from build123d import *

# Parameters (mm, degrees)
ESQUISSE2_W             = 50
ESQUISSE2_H             = 40
BOSS_EXTRU_1_DEPTH      = 5
ESQUISSE3_W             = 73
ESQUISSE3_H             = 38
BOSS_EXTRU_2_DEPTH      = 2.5
ENL_V_MAT_EXTRU_1_REACH = 64.75
ESQUISSE4_R             = 2
ENL_V_MAT_EXTRU_2_REACH = 64.75
ESQUISSE5_W             = 7
ESQUISSE5_H             = 15
CONG_1_R                = 2
CONG_2_R                = 5
CONG_3_R                = 2
ENL_V_MAT_EXTRU_3_DEPTH = 2
ENL_V_MAT_EXTRU_4_REACH = 64.107
ESQUISSE7_R             = 3.5
ENL_V_MAT_EXTRU_5_REACH = 61.643
ESQUISSE8_R             = 2


with BuildPart() as part:
    # Esquisse2 → Boss.-Extru.1 (new body)
    with BuildSketch(Plane(origin=(0, 0, 0), x_dir=(1, 0, 0), z_dir=(0, 1, 0))):
        Rectangle(ESQUISSE2_W, ESQUISSE2_H)
    extrude(amount=BOSS_EXTRU_1_DEPTH)

    # Esquisse3 → Boss.-Extru.2 (add, symmetric)
    with BuildSketch(Plane(origin=(0, 0, 0), x_dir=(0, 0, -1), z_dir=(1, 0, 0))):
        with Locations((0, 24)):
            Rectangle(ESQUISSE3_W, ESQUISSE3_H)
    extrude(amount=BOSS_EXTRU_2_DEPTH, both=True)

    # Esquisse4 → Enl_v. mat.-Extru.1 (cut, up to next)
    with BuildSketch(Plane(origin=(2.5, 0, 0), x_dir=(0, 0, -1), z_dir=(1, 0, 0)), mode=Mode.PRIVATE) as enl_v_mat_extru_1_sk1:
        with Locations((-27.94, 37.97)):
            Circle(ESQUISSE4_R)
    enl_v_mat_extru_1_tool1 = extrude(enl_v_mat_extru_1_sk1.sketch, amount=-ENL_V_MAT_EXTRU_1_REACH, mode=Mode.PRIVATE) & part.part
    # Esquisse4 → Enl_v. mat.-Extru.1 (cut, up to next)
    with BuildSketch(Plane(origin=(2.5, 0, 0), x_dir=(0, 0, -1), z_dir=(1, 0, 0)), mode=Mode.PRIVATE) as enl_v_mat_extru_1_sk2:
        with Locations((-27.94, 10.03)):
            Circle(ESQUISSE4_R)
    enl_v_mat_extru_1_tool2 = extrude(enl_v_mat_extru_1_sk2.sketch, amount=-ENL_V_MAT_EXTRU_1_REACH, mode=Mode.PRIVATE) & part.part
    # Esquisse4 → Enl_v. mat.-Extru.1 (cut, up to next)
    with BuildSketch(Plane(origin=(2.5, 0, 0), x_dir=(0, 0, -1), z_dir=(1, 0, 0)), mode=Mode.PRIVATE) as enl_v_mat_extru_1_sk3:
        with Locations((27.94, 37.97)):
            Circle(ESQUISSE4_R)
    enl_v_mat_extru_1_tool3 = extrude(enl_v_mat_extru_1_sk3.sketch, amount=-ENL_V_MAT_EXTRU_1_REACH, mode=Mode.PRIVATE) & part.part
    # Esquisse4 → Enl_v. mat.-Extru.1 (cut, up to next)
    with BuildSketch(Plane(origin=(2.5, 0, 0), x_dir=(0, 0, -1), z_dir=(1, 0, 0)), mode=Mode.PRIVATE) as enl_v_mat_extru_1_sk4:
        with Locations((27.94, 10.03)):
            Circle(ESQUISSE4_R)
    enl_v_mat_extru_1_tool4 = extrude(enl_v_mat_extru_1_sk4.sketch, amount=-ENL_V_MAT_EXTRU_1_REACH, mode=Mode.PRIVATE) & part.part
    add(enl_v_mat_extru_1_tool1.solids().sort_by_distance((2.5, 37.97, 27.94))[0], mode=Mode.SUBTRACT)
    add(enl_v_mat_extru_1_tool2.solids().sort_by_distance((2.5, 10.03, 27.94))[0], mode=Mode.SUBTRACT)
    add(enl_v_mat_extru_1_tool3.solids().sort_by_distance((2.5, 37.97, -27.94))[0], mode=Mode.SUBTRACT)
    add(enl_v_mat_extru_1_tool4.solids().sort_by_distance((2.5, 10.03, -27.94))[0], mode=Mode.SUBTRACT)

    # Esquisse5 → Enl_v. mat.-Extru.2 (cut, up to next)
    with BuildSketch(Plane(origin=(2.5, 0, 0), x_dir=(0, 0, -1), z_dir=(1, 0, 0)), mode=Mode.PRIVATE) as enl_v_mat_extru_2_sk1:
        with Locations((-33, 24)):
            Rectangle(ESQUISSE5_W, ESQUISSE5_H)
    enl_v_mat_extru_2_tool1 = extrude(enl_v_mat_extru_2_sk1.sketch, amount=-ENL_V_MAT_EXTRU_2_REACH, mode=Mode.PRIVATE) & part.part
    # Esquisse5 → Enl_v. mat.-Extru.2 (cut, up to next)
    with BuildSketch(Plane(origin=(2.5, 0, 0), x_dir=(0, 0, -1), z_dir=(1, 0, 0)), mode=Mode.PRIVATE) as enl_v_mat_extru_2_sk2:
        with Locations((33, 24)):
            Rectangle(ESQUISSE5_W, ESQUISSE5_H)
    enl_v_mat_extru_2_tool2 = extrude(enl_v_mat_extru_2_sk2.sketch, amount=-ENL_V_MAT_EXTRU_2_REACH, mode=Mode.PRIVATE) & part.part
    add(enl_v_mat_extru_2_tool1.solids().sort_by_distance((2.5, 24, 33))[0], mode=Mode.SUBTRACT)
    add(enl_v_mat_extru_2_tool2.solids().sort_by_distance((2.5, 24, -33))[0], mode=Mode.SUBTRACT)

    # Cong_1
    cong_1_edges = [part.edges().sort_by_distance(p)[0] for p in [
        (0, 16.5, -29.5),
        (0, 31.5, -29.5),
        (0, 16.5, 29.5),
        (0, 31.5, 29.5),
        (-2.5, 5, 0),
        (2.5, 5, 0),
    ]]
    fillet(cong_1_edges, radius=CONG_1_R)
    cong_1_2_edges = [part.edges().sort_by_distance(p)[0] for p in [
        (0, 5, -36.5),
        (0, 16.5, -36.5),
        (0, 43, -36.5),
        (0, 31.5, -36.5),
        (0, 5, 36.5),
        (0, 16.5, 36.5),
        (0, 31.5, 36.5),
        (0, 43, 36.5),
    ]]
    fillet(cong_1_2_edges, radius=CONG_1_R)

    # Cong_2
    cong_2_edges = [part.edges().sort_by_distance(p)[0] for p in [
        (25, 2.5, 20),
        (-25, 2.5, 20),
        (-25, 2.5, -20),
        (25, 2.5, -20),
    ]]
    fillet(cong_2_edges, radius=CONG_2_R)

    # Cong_3
    cong_3_edges = [part.edges().sort_by_distance(p)[0] for p in [
        (-2.5, 6, 20),
        (2.5, 6, 20),
        (0, 5, 20),
        (2.5, 6, -20),
        (-2.5, 6, -20),
        (0, 5, -20),
    ]]
    fillet(cong_3_edges, radius=CONG_3_R - 0.0001)  # a hair under: the kernel refuses the full size

    # Esquisse6 → Enl_v. mat.-Extru.3 (cut)
    with BuildSketch(Plane(origin=(0, 5, 0), x_dir=(1, 0, 0), z_dir=(0, 1, 0))):
        Polygon((-12.113248654, 10), (-13.556624327, 12.5), (-16.443375673, 12.5), (-17.886751346, 10), (-16.443375673, 7.5), (-13.556624327, 7.5), align=None)
        Polygon((-12.113248654, -10), (-13.556624327, -7.5), (-16.443375673, -7.5), (-17.886751346, -10), (-16.443375673, -12.5), (-13.556624327, -12.5), align=None)
        Polygon((13.556624327, -12.5), (12.113248654, -10), (13.556624327, -7.5), (16.443375673, -7.5), (17.886751346, -10), (16.443375673, -12.5), align=None)
        Polygon((13.556624327, 7.5), (12.113248654, 10), (13.556624327, 12.5), (16.443375673, 12.5), (17.886751346, 10), (16.443375673, 7.5), align=None)
    extrude(amount=-ENL_V_MAT_EXTRU_3_DEPTH, mode=Mode.SUBTRACT)

    # Esquisse7 → Enl_v. mat.-Extru.4 (cut, up to next)
    with BuildSketch(Plane.ZY.offset(1), mode=Mode.PRIVATE) as enl_v_mat_extru_4_sk1:
        with Locations((-27.94, 37.97)):
            Circle(ESQUISSE7_R)
    enl_v_mat_extru_4_tool1 = extrude(enl_v_mat_extru_4_sk1.sketch, amount=ENL_V_MAT_EXTRU_4_REACH, mode=Mode.PRIVATE) & part.part
    # Esquisse7 → Enl_v. mat.-Extru.4 (cut, up to next)
    with BuildSketch(Plane.ZY.offset(1), mode=Mode.PRIVATE) as enl_v_mat_extru_4_sk2:
        with Locations((-27.94, 10.03)):
            Circle(ESQUISSE7_R)
    enl_v_mat_extru_4_tool2 = extrude(enl_v_mat_extru_4_sk2.sketch, amount=ENL_V_MAT_EXTRU_4_REACH, mode=Mode.PRIVATE) & part.part
    # Esquisse7 → Enl_v. mat.-Extru.4 (cut, up to next)
    with BuildSketch(Plane.ZY.offset(1), mode=Mode.PRIVATE) as enl_v_mat_extru_4_sk3:
        with Locations((27.94, 37.97)):
            Circle(ESQUISSE7_R)
    enl_v_mat_extru_4_tool3 = extrude(enl_v_mat_extru_4_sk3.sketch, amount=ENL_V_MAT_EXTRU_4_REACH, mode=Mode.PRIVATE) & part.part
    # Esquisse7 → Enl_v. mat.-Extru.4 (cut, up to next)
    with BuildSketch(Plane.ZY.offset(1), mode=Mode.PRIVATE) as enl_v_mat_extru_4_sk4:
        with Locations((27.94, 10.03)):
            Circle(ESQUISSE7_R)
    enl_v_mat_extru_4_tool4 = extrude(enl_v_mat_extru_4_sk4.sketch, amount=ENL_V_MAT_EXTRU_4_REACH, mode=Mode.PRIVATE) & part.part
    enl_v_mat_extru_4_1 = enl_v_mat_extru_4_tool1.solids().sort_by_distance((-1, 37.97, -27.94))[0]
    add(enl_v_mat_extru_4_1, mode=Mode.SUBTRACT)
    enl_v_mat_extru_4_2 = enl_v_mat_extru_4_tool2.solids().sort_by_distance((-1, 10.03, -27.94))[0]
    add(enl_v_mat_extru_4_2, mode=Mode.SUBTRACT)
    enl_v_mat_extru_4_3 = enl_v_mat_extru_4_tool3.solids().sort_by_distance((-1, 37.97, 27.94))[0]
    add(enl_v_mat_extru_4_3, mode=Mode.SUBTRACT)
    enl_v_mat_extru_4_4 = enl_v_mat_extru_4_tool4.solids().sort_by_distance((-1, 10.03, 27.94))[0]
    add(enl_v_mat_extru_4_4, mode=Mode.SUBTRACT)
    enl_v_mat_extru_4 = enl_v_mat_extru_4_1 + enl_v_mat_extru_4_2 + enl_v_mat_extru_4_3 + enl_v_mat_extru_4_4  # Enl_v. mat.-Extru.4 as one shape, for the pattern or mirror that repeats it

    # Sym_trie3: Enl_v. mat.-Extru.4 across plane
    add(enl_v_mat_extru_4.mirror(Plane(origin=(0, 0, 0), x_dir=(0, 0, 1), z_dir=(1, 0, 0))), mode=Mode.SUBTRACT)

    # Esquisse8 → Enl_v. mat.-Extru.5 (cut, up to next)
    with BuildSketch(Plane(origin=(0, 3, 0), x_dir=(1, 0, 0), z_dir=(0, 1, 0)), mode=Mode.PRIVATE) as enl_v_mat_extru_5_sk1:
        with Locations(Location((-15, 10, 0), (0, 0, 270))):
            Circle(ESQUISSE8_R)
    enl_v_mat_extru_5_tool1 = extrude(enl_v_mat_extru_5_sk1.sketch, amount=-ENL_V_MAT_EXTRU_5_REACH, mode=Mode.PRIVATE) & part.part
    # Esquisse8 → Enl_v. mat.-Extru.5 (cut, up to next)
    with BuildSketch(Plane(origin=(0, 3, 0), x_dir=(1, 0, 0), z_dir=(0, 1, 0)), mode=Mode.PRIVATE) as enl_v_mat_extru_5_sk2:
        with Locations(Location((-15, -10, 0), (0, 0, 270))):
            Circle(ESQUISSE8_R)
    enl_v_mat_extru_5_tool2 = extrude(enl_v_mat_extru_5_sk2.sketch, amount=-ENL_V_MAT_EXTRU_5_REACH, mode=Mode.PRIVATE) & part.part
    # Esquisse8 → Enl_v. mat.-Extru.5 (cut, up to next)
    with BuildSketch(Plane(origin=(0, 3, 0), x_dir=(1, 0, 0), z_dir=(0, 1, 0)), mode=Mode.PRIVATE) as enl_v_mat_extru_5_sk3:
        with Locations(Location((15, -10, 0), (0, 0, 270))):
            Circle(ESQUISSE8_R)
    enl_v_mat_extru_5_tool3 = extrude(enl_v_mat_extru_5_sk3.sketch, amount=-ENL_V_MAT_EXTRU_5_REACH, mode=Mode.PRIVATE) & part.part
    # Esquisse8 → Enl_v. mat.-Extru.5 (cut, up to next)
    with BuildSketch(Plane(origin=(0, 3, 0), x_dir=(1, 0, 0), z_dir=(0, 1, 0)), mode=Mode.PRIVATE) as enl_v_mat_extru_5_sk4:
        with Locations(Location((15, 10, 0), (0, 0, 270))):
            Circle(ESQUISSE8_R)
    enl_v_mat_extru_5_tool4 = extrude(enl_v_mat_extru_5_sk4.sketch, amount=-ENL_V_MAT_EXTRU_5_REACH, mode=Mode.PRIVATE) & part.part
    add(enl_v_mat_extru_5_tool1.solids().sort_by_distance((-15, 3, -10))[0], mode=Mode.SUBTRACT)
    add(enl_v_mat_extru_5_tool2.solids().sort_by_distance((-15, 3, 10))[0], mode=Mode.SUBTRACT)
    add(enl_v_mat_extru_5_tool3.solids().sort_by_distance((15, 3, 10))[0], mode=Mode.SUBTRACT)
    add(enl_v_mat_extru_5_tool4.solids().sort_by_distance((15, 3, -10))[0], mode=Mode.SUBTRACT)


solid = part.part
Could you check a few things on this model? Use its own coordinates, in mm. A direction names the side the tool comes from. Coordinates: 2 decimals unless noted, no trailing zeros. Order: outer loops, then holes, each group sorted by start corner. A loop starts at its lowest first (then second) coordinate and runs counter-clockwise, first axis right, second up. Notation, with made-up numbers: (-12.75, 50.5) - (31.25, 50.5) arc R27 ccw to (31.25, 76.5) - close; hole circle Ø3 at (51.5, 88). An arc over 180 degrees is marked (long way). Answer in a Markdown table with one row per item. Add a question column.
(1) I need wall thicknesses on L1, parallel to Y at x = 1.95, z = -27.94; L2, parallel to Z at x = 1.75, y = 37.97; L3, parallel to X at y = 2.3, z = -10. Which ranges of each line are inside material? Lowest first, please.
(2) If we section it at A-A, the plane x = 15: Please give me the cut outline in (y, z), then the cut area to 3 significant figures.
(3) If we section it at D-D, the plane z = 0.5: Please give me the cut outline in (x, y), then the cut area to 3 significant figures.
(4) Will these pins go through, and if not, where does the flat tip stop? pin 1 (2 mm diameter, centred on x = -15, y = 4, fed in from -Z); pin 2 (8 mm diameter, centred on x = -19.5, z = -18.5, fed in from +Y); pin 3 (6 mm diameter, centred on y = 16.5, z = -28, fed in from -X); pin 4 (3 mm diameter, centred on x = -9.5, z = 20, fed in from -Y).
(5) If we section it at B-B, the plane z = -27.94: Please give me the cut outline in (x, y).
(6) If we mould it in two halves opening along Y, with no side actions, what happens to faces 1 (the face through (0.06, 4.13, -20.35)), 2 (the face through (13, 3, 11)), 3 (the face through (1, 10.1, 30.2)), 4 (the face through (-13, 2, -10))? For each: released by +Y, released by -Y, zero draft, split by the parting line, or undercut.
(7) On a 3-axis mill with a long thin cutter (end or side, diameter ignored), from which of +Z, -Z, +X, -X, +Y, -Y can I reach the whole of each face in a straight line? I mean faces 5 (the face through (15, 5, 0)), 6 (the face through (-15, 4, 12.5)), 7 (the face through (0, 5, -28)), 8 (the face through (0, 24, -29.5)), 9 (the face through (-1, 36, 29)). Say none if no direction works.
(8) If we section it at C-C, the plane y = 10.03: Please give me the cut outline in (x, z), then the cut area to 3 significant figures.
Results are:
| question | item | result |
|---|---|---|
| 1 | L1 | y = 5 to 6.53, 13.53 to 34.47, 41.47 to 43 |
| 1 | L2 | z = -36.5 to -31.44, -24.44 to 24.44, 31.44 to 36.5 |
| 1 | L3 | x = -25 to -17, -13 to 13, 17 to 25 |
| 2 | outline | (0, -20) - (5, -20) - (5, -12.5) - (3, -12.5) - (3, -12) - (0, -12) - close; (0, -8) - (3, -8) - (3, -7.5) - (5, -7.5) - (5, 7.5) - (3, 7.5) - (3, 8) - (0, 8) - close; (0, 12) - (3, 12) - (3, 12.5) - (5, 12.5) - (5, 20) - (0, 20) - close |
| 2 | area | 156 mm2 |
| 3 | outline | (-25, 0) - (25, 0) - (25, 5) - (4.5, 5) arc R2 cw to (2.5, 7) - (2.5, 43) - (-2.5, 43) - (-2.5, 7) arc R2 cw to (-4.5, 5) - (-25, 5) - close |
| 3 | area | 442 mm2 |
| 4 | pin 1 | stops at z = -20 |
| 4 | pin 2 | stops at y = 5 |
| 4 | pin 3 | stops at x = -2.5 |
| 4 | pin 4 | stops at y = 0 |
| 5 | outline | (-2.5, 5) - (2.5, 5) - (2.5, 6.53) - (1, 6.53) - (1, 8.03) - (-1, 8.03) - (-1, 6.53) - (-2.5, 6.53) - close; (-2.5, 13.53) - (-1, 13.53) - (-1, 12.03) - (1, 12.03) - (1, 13.53) - (2.5, 13.53) - (2.5, 34.47) - (1, 34.47) - (1, 35.97) - (-1, 35.97) - (-1, 34.47) - (-2.5, 34.47) - close; (-2.5, 41.47) - (-1, 41.47) - (-1, 39.97) - (1, 39.97) - (1, 41.47) - (2.5, 41.47) - (2.5, 43) - (-2.5, 43) - close |
| 6 | face 1 | released by -Y |
| 6 | face 2 | released by +Y |
| 6 | face 3 | undercut |
| 6 | face 4 | zero draft |
| 7 | face 5 | +Z, -Z, +X, +Y |
| 7 | face 6 | +Y |
| 7 | face 7 | -Z, +X, -X, -Y |
| 7 | face 8 | -Z, +X, -X |
| 7 | face 9 | -X |
| 8 | outline | (-2.5, -36.5) - (2.5, -36.5) - (2.5, -31.44) - (1, -31.44) - (1, -29.94) - (-1, -29.94) - (-1, -31.44) - (-2.5, -31.44) - close; (-2.5, -24.44) - (-1, -24.44) - (-1, -25.94) - (1, -25.94) - (1, -24.44) - (2.5, -24.44) - (2.5, 24.44) - (1, 24.44) - (1, 25.94) - (-1, 25.94) - (-1, 24.44) - (-2.5, 24.44) - close; (-2.5, 31.44) - (-1, 31.44) - (-1, 29.94) - (1, 29.94) - (1, 31.44) - (2.5, 31.44) - (2.5, 36.5) - (-2.5, 36.5) - close |
| 8 | area | 307 mm2 |
